from build123d import *

# Parameters (mm, degrees)
SKETCH1_W           = 52
SKETCH1_H           = 24
SKETCH1_R           = 8.25
BOSS_EXTRUDE1_DEPTH = 12
SKETCH2_R           = 1
CUT_EXTRUDE1_DEPTH  = 32.048349393
SKETCH3_R           = 1.75
CUT_EXTRUDE2_DEPTH  = 1
CUT_EXTRUDE3_DEPTH  = 5
FILLET3_R           = 0.5
CHAMFER1_SIZE       = 2.5


with BuildPart() as part:
    # Sketch1 → Boss-Extrude1 (new body)
    with BuildSketch(Plane(origin=(0, 0, 0), x_dir=(1, 0, 0), z_dir=(0, 1, 0))):
        Rectangle(SKETCH1_W, SKETCH1_H)
        with Locations(Location((12.75, 0, 0), (0, 0, 270))):
            Circle(SKETCH1_R, mode=Mode.SUBTRACT)
        with Locations(Location((-12.75, 0, 0), (0, 0, 270))):
            Circle(SKETCH1_R, mode=Mode.SUBTRACT)
    extrude(amount=BOSS_EXTRUDE1_DEPTH)

    # Sketch2 → Cut-Extrude1 (cut, through all)
    with BuildSketch(Plane(origin=(0, 12, 0), x_dir=(1, 0, 0), z_dir=(0, 1, 0))):
        with Locations(Location((-21.35, 8.85, 0), (0, 0, 270))):
            Circle(SKETCH2_R)
        with Locations(Location((21.35, 8.85, 0), (0, 0, 270))):
            Circle(SKETCH2_R)
        with Locations(Location((21.35, -8.85, 0), (0, 0, 270))):
            Circle(SKETCH2_R)
        with Locations(Location((-21.35, -8.85, 0), (0, 0, 270))):
            Circle(SKETCH2_R)
    extrude(amount=-CUT_EXTRUDE1_DEPTH, mode=Mode.SUBTRACT)

    # Sketch3 → Cut-Extrude2 (cut)
    with BuildSketch(Plane(origin=(0, 12, 0), x_dir=(1, 0, 0), z_dir=(0, 1, 0))):
        with Locations(Location((-21.35, 8.85, 0), (0, 0, 270))):
            Circle(SKETCH3_R)
        with Locations(Location((21.35, 8.85, 0), (0, 0, 270))):
            Circle(SKETCH3_R)
        with Locations(Location((21.35, -8.85, 0), (0, 0, 270))):
            Circle(SKETCH3_R)
        with Locations(Location((-21.35, -8.85, 0), (0, 0, 270))):
            Circle(SKETCH3_R)
    extrude(amount=-CUT_EXTRUDE2_DEPTH, mode=Mode.SUBTRACT)

    # Sketch4 → Cut-Extrude3 (cut)
    with BuildSketch(Plane.XZ):
        Polygon((-6, -5), (-6, -12), (6, -12), (6, -5), (0, -5), align=None)
    extrude(amount=-CUT_EXTRUDE3_DEPTH, mode=Mode.SUBTRACT)

    # Fillet3
    fillet3_edges = [part.edges().sort_by_distance(p)[0] for p in [
        (-6, 2.5, -5),
        (6, 5, -8.5),
        (6, 2.5, -5),
        (-6, 5, -8.5),
        (0, 5, -5),
    ]]
    fillet(fillet3_edges, radius=FILLET3_R)

    # Chamfer1
    chamfer1_edges = [part.edges().sort_by_distance(p)[0] for p in [
        (26, 6, 12),
        (-26, 6, 12),
        (-26, 6, -12),
        (26, 6, -12),
    ]]
    chamfer(chamfer1_edges, length=CHAMFER1_SIZE)


solid = part.part
Geometry check sheet. Reference: the model listing, model coordinates, mm. A direction names the side the tool comes from. Give positions to 0.01 mm unless a question says otherwise; leave off trailing zeros. Order: outer loops, then holes, each group sorted by start corner. A loop starts at its lowest first (then second) coordinate and runs counter-clockwise, first axis right, second up.
1) Cross-section at B-B (z = 0). Record the boundary of the cut face in (x, y).
Results are:
outline: (-26, 0) - (-21, 0) - (-21, 12) - (-26, 12) - close; (-4.5, 0) - (4.5, 0) - (4.5, 12) - (-4.5, 12) - close; (21, 0) - (26, 0) - (26, 12) - (21, 12) - close
2) Tool access check on faces 1 (the flat face through (0, 2, -5)), 2 (the cylindrical face through (19.8, 11.51, 9.66)), 3 (the cylindrical face through (-15.91, 5.92, 7.62)). Record the directions out of +Z, -Z, +X, -X, +Y, -Y that give a thin tool (end or side, any length) a straight path to the whole face; none if there is none.
Results are:
face 1: -Z, -Y
face 2: +Y
face 3: +Y, -Y
3) Cross-section at D-D (x = 4). Record the boundary of the cut face in (y, z).
Results are:
outline: (0, -5) - (4.5, -5) arc R0.5 cw to (5, -5.5) - (5, -12) - (12, -12) - (12, 12) - (0, 12) - close
4) Gauge pin test, flat ends, axial feed: pin 1 (4 mm diameter, centred on x = 21.35, z = 8.85, fed in from -Y); pin 2 (2 mm diameter, centred on x = 1.5, y = 2, fed in from -Z). Record the tip position at first contact, or that the pin passes through.
Results are:
pin 1: stops at y = 0
pin 2: stops at z = -5
5) Cross-section at A-A (x = -12.75). Record the boundary of the cut face in (y, z).
Results are:
outline: (0, -12) - (12, -12) - (12, -8.25) - (0, -8.25) - close; (0, 8.25) - (12, 8.25) - (12, 12) - (0, 12) - close
6) Material ranges on probe 1 along X at (y, z) = (3, 8.85); probe 2 along X at (y, z) = (2.75, -8.85); probe 3 along X at (y, z) = (6, 0), recorded low to high.
Results are:
probe 1: x = -26 to -22.35, -20.35 to 20.35, 22.35 to 26
probe 2: x = -26 to -22.35, -20.35 to -6, 6 to 20.35, 22.35 to 26
probe 3: x = -26 to -21, -4.5 to 4.5, 21 to 26
7) Draft check along Z on faces 4 (the cylindrical face through (-23.06, 11.51, 8.47)), 5 (the flat face through (0, 6, 12)), 6 (the flat face through (0, 0, 0)). Enter one of: released by +Z, released by -Z, zero draft, split by the parting line, or undercut.
Results are:
face 4: undercut
face 5: released by +Z
face 6: zero draft
8) Cross-section at C-C (y = 6.25). Record the boundary of the cut face in (x, z), then the cut area to 3 significant figures.
Results are:
outline: (-26, -9.5) - (-23.5, -12) - (23.5, -12) - (26, -9.5) - (26, 9.5) - (23.5, 12) - (-23.5, 12) - (-26, 9.5) - close; hole circle Ø2 at (-21.35, -8.85); hole circle Ø2 at (-21.35, 8.85); hole circle Ø16.5 at (-12.75, 0); hole circle Ø16.5 at (12.75, 0); hole circle Ø2 at (21.35, -8.85); hole circle Ø2 at (21.35, 8.85)
area: 795 mm2
